Verification items for the finished model (mm, model axes). Face numbers are marked on the shaded views. A direction names the side the tool comes from. Give positions to 0.01 mm unless a question says otherwise; leave off trailing zeros. Write each loop counter-clockwise with the first axis right and the second up, starting at its lowest first coordinate (ties: lowest second). Pieces come first, ordered by that corner, then holes. Notation, with made-up numbers: (50, -16.75) - (84, -16.75) arc R26 cw to (84, 1.25) - close; hole circle Ø6 at (-29, 12.25). An arc over 180 degrees is marked (long way). Put each result on its own line as item: value.
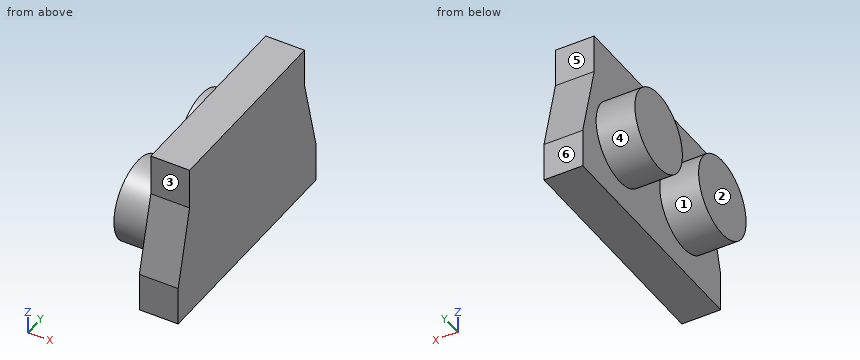
from build123d import *

# Parameters (mm, degrees)
F1_DEPTH = 25.4
F2_R     = 26.2509
F3_DEPTH = 25.4


with BuildPart() as f1:
    # F0 (on Right) → F1 (new body)
    with BuildSketch(Plane.YZ):
        Polygon((-76.2, -42.571535), (76.2, -42.571535), (76.2, -17.171535), (63.5, -17.171535), (-63.5, -17.171535), (-76.2, -17.171535), align=None)
        Polygon((63.5, -17.171535), (76.2, -17.171535), (63.5, 33.628465), (63.5, 59.028465), (-63.5, 59.028465), (-63.5, 32.015353), (-76.2, -17.171535), (-63.5, -17.171535), align=None)
    extrude(amount=F1_DEPTH)

    # F2 (on Right) → F3 (join)
    with BuildSketch(Plane.YZ):
        with Locations((35.200721, 0)):
            Circle(F2_R)
        with Locations((-35.200721, 0)):
            Circle(F2_R)
    extrude(amount=-F3_DEPTH)


solid = f1.part
Q1. Section check C-C, the plane z = 3. Record the cut outline in (x, y).
Answers follow:
outline: (-25.4, -61.28) - (0, -61.28) - (0, -70.99) - (25.4, -70.99) - (25.4, 71.16) - (0, 71.16) - (0, 61.28) - (-25.4, 61.28) - (-25.4, 9.12) - (0, 9.12) - (0, -9.12) - (-25.4, -9.12) - close
Q2. Section check D-D, the plane y = -11. Record the cut outline in (x, z).
Answers follow:
outline: (-25.4, -10.17) - (0, -10.17) - (0, -42.57) - (25.4, -42.57) - (25.4, 59.03) - (0, 59.03) - (0, 10.17) - (-25.4, 10.17) - close
Q3. Set-up check for the marked faces 4, 5 and 6: record each of +Z, -Z, +X, -X, +Y, -Y from which the full face is reachable in a straight line by a thin tool's end or side.
Answers follow:
face 4: -X
face 5: +Z, +X, -X, +Y
face 6: +Z, -Z, +X, -X, +Y
Q4. Section check B-B, the plane x = -11. Record the cut outline in (y, z), plus the area to 3 significant figures.
Answers follow:
outline: circle Ø52.5 at (-35.2, 0); circle Ø52.5 at (35.2, 0)
area: 4,330 mm2
Q5. Section check A-A, the plane x = 20.5. Record the cut outline in (y, z), plus the area to 3 significant figures.
Answers follow:
outline: (-76.2, -42.57) - (76.2, -42.57) - (76.2, -17.17) - (63.5, 33.63) - (63.5, 59.03) - (-63.5, 59.03) - (-63.5, 32.02) - (-76.2, -17.17) - close
area: 14,200 mm2
Q6. Go/stop test with flat-tipped pins: pin 1 Ø12 at (x, z) = (-9, -3.5) entering from +Y; pin 2 Ø10 at (x, z) = (18.5, 30) entering from +Y; pin 3 Ø1.5 at (y, z) = (-10.5, 17.5) entering from -X; pin 4 Ø12 at (x, y) = (-3.5, 46.5) entering from +Z. Record where each tip stops, or that it passes through.
Answers follow:
pin 1: stops at y = 61.45
pin 2: stops at y = 65.66
pin 3: stops at x = 0
pin 4: stops at z = 59.03
Q7. Scan lines: line 1 along Y through (x, z) = (17.5, 35); line 2 along X through (y, z) = (45, 27); line 3 along Y through (x, z) = (-21.5, -10). Record each from-to range of solid material in increasing order.
Answers follow:
line 1: y = -63.5 to 63.5
line 2: x = 0 to 25.4
line 3: y = -59.47 to -10.93, 10.93 to 59.47
Q8. Release check for a two-part mould opening along Y. For the marked faces 1, 2 and 3 record: released by +Y, released by -Y, zero draft, split by the parting line, or undercut.
Answers follow:
face 1: undercut
face 2: zero draft
face 3: released by -Y
